from build123d import *

# Parameters (mm, degrees)
ESQUISSE1_W             = 85
ESQUISSE1_H             = 72
BOSS_EXTRU_1_DEPTH      = 2
BOSS_EXTRU_2_DEPTH      = 3
ESQUISSE3_R             = 3.75
ESQUISSE3_R_2           = 3
ENL_V_MAT_EXTRU_1_DEPTH = 56.921820428
ESQUISSE4_R             = 6
ESQUISSE4_R_2           = 3.5
ENL_V_MAT_EXTRU_2_DEPTH = 2
ESQUISSE8_W             = 7
ESQUISSE8_H             = 2.25
BOSS_EXTRU_4_DEPTH      = 12
CONG_4_R                = 2


with BuildPart() as part:
    # Esquisse1 → Boss.-Extru.1 (new body)
    with BuildSketch(Plane(origin=(0, 0, 0), x_dir=(1, 0, 0), z_dir=(0, 1, 0))):
        Rectangle(ESQUISSE1_W, ESQUISSE1_H)
    extrude(amount=BOSS_EXTRU_1_DEPTH)

    # Esquisse2 → Boss.-Extru.2 (add)
    with BuildSketch(Plane(origin=(0, 2, 0), x_dir=(1, 0, 0), z_dir=(0, 1, 0))):
        Polygon((40.25, -33.75), (-40.25, -33.75), (-40.25, 17.75), (-24.25, 17.75), (-24.25, 33.75), (40.25, 33.75), align=None)
        Polygon((-38.25, -31.75), (38.25, -31.75), (38.25, 31.75), (-22.25, 31.75), (-22.25, 15.75), (-38.25, 15.75), align=None, mode=Mode.SUBTRACT)
    extrude(amount=BOSS_EXTRU_2_DEPTH)

    # Esquisse3 → Enlèv. mat.-Extru.1 (cut, through all)
    with BuildSketch(Plane(origin=(0, 0, 0), x_dir=(-1, 0, 0), z_dir=(0, -1, 0))):
        with Locations(Location((-22.5, -28.5, 0), (0, 0, 90))):
            Circle(ESQUISSE3_R)
        with Locations(Location((-7.5, -28.5, 0), (0, 0, 90))):
            Circle(ESQUISSE3_R)
        with Locations(Location((7.5, -28.5, 0), (0, 0, 90))):
            Circle(ESQUISSE3_R_2)
    extrude(amount=-ENL_V_MAT_EXTRU_1_DEPTH, mode=Mode.SUBTRACT)

    # Esquisse4 → Enlèv. mat.-Extru.2 (cut)
    with BuildSketch(Plane(origin=(0, 0, 0), x_dir=(-1, 0, 0), z_dir=(0, -1, 0))):
        with Locations(Location((-27.5, 21, 0), (0, 0, 90))):
            Circle(ESQUISSE4_R)
        with Locations(Location((7.5, 21, 0), (0, 0, 90))):
            Circle(ESQUISSE4_R_2)
    extrude(amount=-ENL_V_MAT_EXTRU_2_DEPTH, mode=Mode.SUBTRACT)

    # Esquisse8 → Boss.-Extru.4 (add)
    with BuildSketch(Plane(origin=(0, 2, 0), x_dir=(1, 0, 0), z_dir=(0, 1, 0))):
        with Locations((-27, -34.875)):
            Rectangle(ESQUISSE8_W, ESQUISSE8_H)
    extrude(amount=BOSS_EXTRU_4_DEPTH)

    # Congé4
    cong_4_edges = [part.edges().sort_by_distance(p)[0] for p in [
        (0, 0, -36),
        (42.5, 0, 0),
        (0, 0, 36),
        (-42.5, 0, 0),
        (-42.5, 1, -36),
        (42.5, 1, -36),
        (42.5, 1, 36),
        (-42.5, 1, 36),
    ]]
    fillet(cong_4_edges, radius=CONG_4_R - 0.0001)  # a hair under: the kernel refuses the full size


solid = part.part
Work out the finished part from the listing and answer in its coordinate system (mm). A direction names the side the tool comes from. Round coordinates to 2 decimals unless told otherwise and drop trailing zeros.
1) A tool of negligible diameter and unlimited length cuts with its end or side. For faces 1 (the cylindrical face through (0.57, 0.6, -35.43)), 2 (the flat face through (-24.25, 3, -26)), 3 (the flat face through (-30, 3, -15.75)), 4 (the cylindrical face through (-7.4, 1, 31.5)), 5 (the flat face through (9, 3, 33.75)), from which of +Z, -Z, +X, -X, +Y, -Y can it reach the whole face along a straight path? Write none if from no direction.
2) A cutting plane is placed at A-A (z = 28.5). Give the number of separate pieces and of enclosed holes in the cut face, plus the area to 3 significant figures.
3) Straight lines are drawn through the part: line 1 (X direction, y = 0.4, z = -21); line 2 (Z direction, x = 7.5, y = 2.7); line 3 (X direction, y = 1.65, z = -21). For each, find the intervals that lie inside material, in ascending order.
4) The mould has two halves that part along Z. Classify faces 6 (the flat face through (-40.25, 3, 8)), 7 (the cylindrical face through (-8.841, 0.986, -24.233)), 8 (the cylindrical face through (0.57, 0.6, 35.43)): pulls with the +Z half, pulls with the -Z half, needs draft (parallel to the pull), parting line crosses it, or undercut.
5) Given pin 1 Ø11 at (x, z) = (27.5, -21) entering from -Y; pin 2 Ø1.5 at (x, z) = (-27.5, 10) entering from +Y; pin 3 Ø1.5 at (x, y) = (29.5, 4) entering from -Z; pin 4 Ø1.1 at (y, z) = (5, 35.5) entering from -X, each flat-ended and moving along its own axis, determine where each tip first touches the part or whether it passes through.
Completed:
1. face 1: -Z, +X, -X, -Y
1. face 2: -Z, -X, +Y
1. face 3: +Y
1. face 4: +Y, -Y
1. face 5: +Z, +X, +Y
2. separate pieces: 4
2. enclosed holes: 0
2. area: 138 mm2
3. line 1: x = -41.7 to -11, -4 to 21.5, 33.5 to 41.7
3. line 2: z = -33.75 to -31.75, 32.25 to 33.75
3. line 3: x = -42.47 to -11, -4 to 21.5, 33.5 to 42.47
4. face 6: needs draft
4. face 7: undercut
4. face 8: pulls with the +Z half
5. pin 1: passes through
5. pin 2: stops at y = 2
5. pin 3: stops at z = -33.75
5. pin 4: stops at x = -30.5
